from build123d import *

# Parameters (mm, degrees)
SKETCH1_W          = 6
SKETCH1_H          = 1
CHAMFER1_SIZE      = 0.3
CUT_EXTRUDE2_DEPTH = 0.84


with BuildPart() as part:
    # Sketch1 → Revolve1 (revolve)
    with BuildSketch(Plane(origin=(0, 0, 0), x_dir=(0, 0, -1), z_dir=(1, 0, 0))):
        with Locations((3, 0.5)):
            Rectangle(SKETCH1_W, SKETCH1_H)
    revolve(axis=Axis((0, 0, -6), (0, 0, 1)))

    # Chamfer1
    chamfer1_edges = [part.edges().sort_by_distance(p)[0] for p in [
        (0, -1, -6),
    ]]
    chamfer(chamfer1_edges, length=CHAMFER1_SIZE)

    # Sketch7 → Revolve2 (revolve)
    with BuildSketch(Plane(origin=(0, 0, 0), x_dir=(0, 0, -1), z_dir=(1, 0, 0)), mode=Mode.PRIVATE) as revolve2_sk:
        Polygon((0, 2), (0.2, 2), (1.2, 1), (1.2, 0), (0, 0), align=None)
    revolve(revolve2_sk.sketch.rotate(Axis((0, 0, 0), (0, 0, -1)), 180), axis=Axis((0, 0, 0), (0, 0, -1)))

    # Boss-Extrude1 cone 1 section (through the dimple's axis) → Boss-Extrude1 (revolve)
    with BuildSketch(Plane(origin=(0, 0, -1.2), x_dir=(0, -1, 0), z_dir=(1, 0, 0))):
        Polygon((0, 0), (1, 0), (0, 1), align=None)
    revolve(axis=Axis((0, 0, -1.2), (0, 0, -1)))

    # Sketch5 → Cut-Extrude2 (cut)
    with BuildSketch(Plane.XY):
        Polygon((0.65, -0.375277675), (0.65, 0.375277675), (0, 0.75055535), (-0.65, 0.375277675), (-0.65, -0.375277675), (0, -0.75055535), align=None)
    extrude(amount=-CUT_EXTRUDE2_DEPTH, mode=Mode.SUBTRACT)

    # Cut-Extrude3 cone 1 section (through the dimple's axis) → Cut-Extrude3 (revolve, cut)
    with BuildSketch(Plane(origin=(0, 0, 0), x_dir=(0, -1, 0), z_dir=(1, 0, 0))):
        Polygon((0, 0), (0.75055535, 0), (0, 0.75055535), align=None)
    revolve(axis=Axis((0, 0, 0), (0, 0, -1)), mode=Mode.SUBTRACT)


solid = part.part
Geometry: final body of the model. Coordinates: model frame, mm. Round coordinates to 2 decimals unless told otherwise and drop trailing zeros. Order: outer loops, then holes, each group sorted by start corner. A loop starts at its lowest first (then second) coordinate and runs counter-clockwise, first axis right, second up. Notation, with made-up numbers: (55.5, 46) -> (76.5, 46) arc R23 cw to (76.5, 71) -> close; hole circle Ø5 at (45, -4). An arc over 180 degrees is marked (long way). Put each result on its own line as item: value. Start each with the question number.
Q1. First-contact query: pin 1 (1 mm diameter, centred on y = 1, z = -2, fed in from -X); pin 2 (0.7 mm diameter, centred on x = 0, y = 0, fed in from +Z). Flat tips, straight axial feed; report the tip coordinate or a pass-through.
Q2. Line query: probe 1 along Z at (x, y) = (-0.6, 0); probe 2 along X at (y, z) = (0.4, -0.5); probe 3 along Y at (x, z) = (0.35, -0.5). Output: solid intervals per line, ascending.
Q3. Section B-B on z = -2.6. Return the cut outline in (x, y), and give its area (3 significant figures).
Q4. Section A-A on y = 0. Return the cut outline in (x, z).
Q5. Pull-direction query (X, two-part tool) for faces 1 (the cylindrical face through (1, 0, -3)), 2 (the flat face through (0, 0, -0.84)), 3 (the flat face through (0, 0, -6)); classes: +X half, -X half, draft (parallel to the pull), parting line (faces both ways), or undercut.
Ans:
1. pin 1: stops at x = -0.87
1. pin 2: stops at z = -0.84
2. probe 1: z = -6 to -0.84
2. probe 2: x = -1.65 to -0.61, 0.61 to 1.65
2. probe 3: y = -1.66 to -0.55, 0.55 to 1.66
3. outline: circle Ø2 at (0, 0)
3. area: 3.14 mm2
4. outline: (-2, -0.2) -> (-1, -1.2) -> (-1, -5.7) -> (-0.7, -6) -> (0.7, -6) -> (1, -5.7) -> (1, -1.2) -> (2, -0.2) -> (2, 0) -> (0.75, 0) -> (0.65, -0.1) -> (0.65, -0.84) -> (-0.65, -0.84) -> (-0.65, -0.1) -> (-0.75, 0) -> (-2, 0) -> close
5. face 1: parting line
5. face 2: undercut
5. face 3: draft
